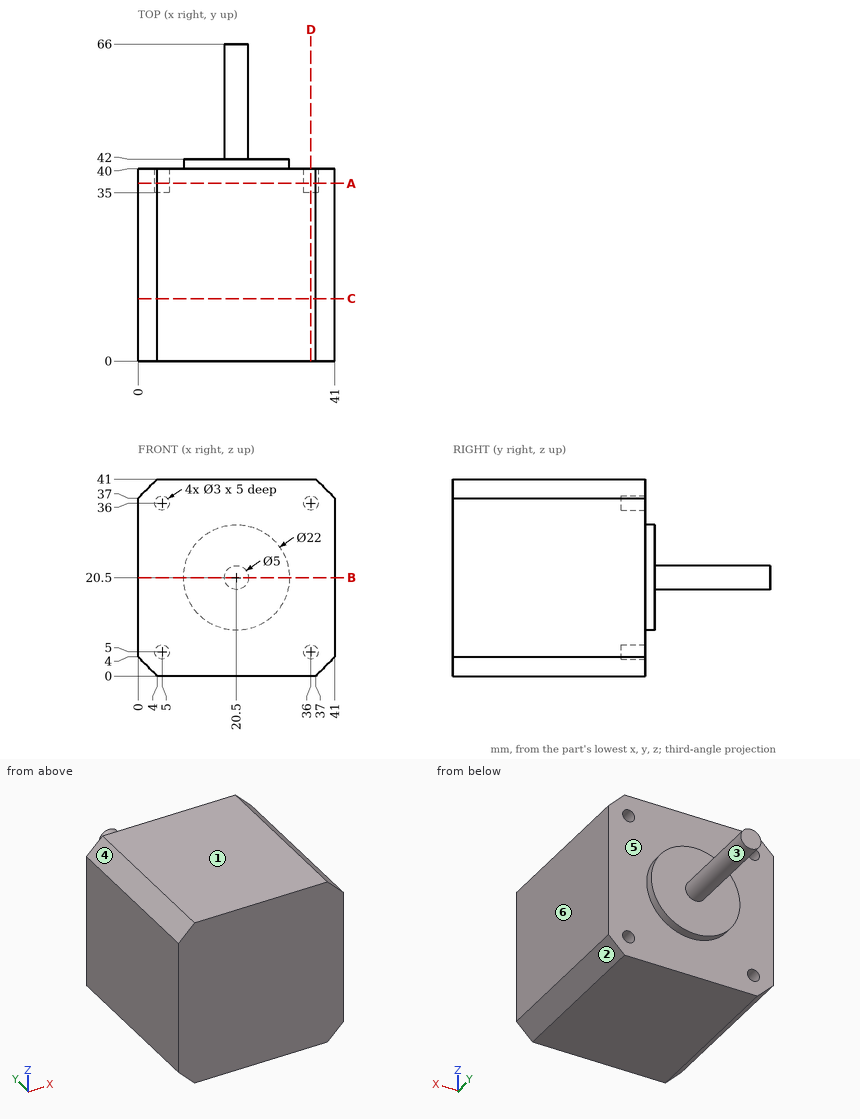
Can you work these out from the drawing? Everything is in mm from the part's minimum corner. A direction names the side the tool comes from. Round coordinates to 2 decimals unless told otherwise and drop trailing zeros. Write each loop counter-clockwise with the first axis right and the second up, starting at its lowest first coordinate (ties: lowest second). Pieces come first, ordered by that corner, then holes. Notation, with made-up numbers: M 3.5,76.5 L 27.5,76.5 A18 ccw 27.5,86.5 Z; hole C 22.5,16.25 d8. An arc over 180 degrees is marked long. Use a Markdown table: item, result.
Item 1: Which directions (+Z, -Z, +X, -X, +Y, -Y) give clear straight access to the entire face, cutting with the end or side of a thin tool? Please do the marked faces 5 and 6.
Found:
| item | result |
|---|---|
| face 5 | +Y |
| face 6 | +Z, -Z, +X, +Y, -Y |
Item 2: I want a section at B-B (z = 20.5). List the corners of the cut face in (x, y) for me, and give its area (3 significant figures).
Found:
| item | result |
|---|---|
| outline | M 0,0 L 41,0 L 41,40 L 31.5,40 L 31.5,42 L 23,42 L 23,66 L 18,66 L 18,42 L 9.5,42 L 9.5,40 L 0,40 Z |
| area | 1,800 mm2 |
Item 3: I want a section at C-C (y = 13). List the corners of the cut face in (x, z) for me.
Found:
| item | result |
|---|---|
| outline | M 0,4 L 4,0 L 37,0 L 41,4 L 41,37 L 37,41 L 4,41 L 0,37 Z |
Item 4: We'd pull the mould along X, two halves only. Please class the marked faces 1, 2, 3 and 4: released by +X, released by -X, zero draft, split by the parting line, or undercut.
Found:
| item | result |
|---|---|
| face 1 | zero draft |
| face 2 | released by +X |
| face 3 | split by the parting line |
| face 4 | released by -X |
Item 5: If I drill on line 1 along Z through (x, y) = (36, 37); line 2 along Y through (x, z) = (20, 38.5), over which ranges is the centre line in solid material (lowest first)? Write a range as [from, to].
Found:
| item | result |
|---|---|
| line 1 | z = [0, 3.5], [6.5, 34.5], [37.5, 41] |
| line 2 | y = [0, 40] |
Item 6: I want a section at D-D (x = 36). List the corners of the cut face in (y, z) for me.
Found:
| item | result |
|---|---|
| outline | M 0,0 L 40,0 L 40,3.5 L 35,3.5 L 35,6.5 L 40,6.5 L 40,34.5 L 35,34.5 L 35,37.5 L 40,37.5 L 40,41 L 0,41 Z |
Item 7: I want a section at A-A (y = 37). List the corners of the cut face in (x, z) for me, and give its area (3 significant figures).
Found:
| item | result |
|---|---|
| outline | M 0,4 L 4,0 L 37,0 L 41,4 L 41,37 L 37,41 L 4,41 L 0,37 Z; hole C 5,5 d3; hole C 5,36 d3; hole C 36,5 d3; hole C 36,36 d3 |
| area | 1,620 mm2 |
Item 8: For pin 1 Ø1.5 at (x, z) = (5.5, 35.5) entering from +Y; pin 2 Ø12 at (y, z) = (49.5, 10.5) entering from -X; pin 3 Ø5 at (x, z) = (36, 5) entering from +Y; pin 4 Ø12 at (x, z) = (24, 35.5) entering from +Y, each with a flat end and sliding along its axis, tell me the tip position at first contact or that it passes through.
Found:
| item | result |
|---|---|
| pin 1 | stops at y = 35 |
| pin 2 | passes through |
| pin 3 | stops at y = 40 |
| pin 4 | stops at y = 42 |
